For this review, take the finished solid that the model builds, in its own axes (mm). Face numbers are marked on the shaded views. A direction names the side the tool comes from. Give positions to 0.01 mm unless a question says otherwise; leave off trailing zeros. Loops run counter-clockwise (first coordinate to the right, second up) from the corner with the lowest first, then second, coordinate; pieces in that order, holes last. Notation, with made-up numbers: (39, 64) - (87, 64) arc R17 ccw to (87, 82) - close; hole circle Ø5 at (57.5, 20). An arc over 180 degrees is marked (long way). Use CSV: the item, a comma, the result in double quotes. Start each with the question number.
1. Take a section at B-B on y = 0. Give the boundary of the cut face in (x, z).
2. Wall thickness on line 1 (Y direction, x = 0, z = 15.2); line 2 (Y direction, x = 0, z = 9.75); line 3 (X direction, y = 2, z = 15.75): over which ranges is each line inside the solid? List them lowest first.
3. For the marked faces 1, 2 and 3, list the 3-axis set-ups (+Z, -Z, +X, -X, +Y, -Y) from which the entire face can be reached by the end or side of a thin tool; tool diameter is ignored.
4. Take a section at C-C on z = 13. Give the boundary of the cut face in (x, y), plus the area to 3 significant figures.
5. Mouldability with a two-part tool opening along Y and no side actions: class the marked faces 4, 5 and 6 as pulls with the +Y half, pulls with the -Y half, needs draft (parallel to the pull), parting line crosses it, or undercut.
6. Take a section at A-A on x = 0. Give the boundary of the cut face in (y, z), plus the area to 3 significant figures.
7. For pin 1 (2 mm diameter, centred on y = 20.5, z = 7.5, fed in from +X); pin 2 (5 mm diameter, centred on y = -5, z = 11, fed in from +X); pin 3 (8 mm diameter, centred on x = 9.5, z = 6.5, fed in from +Y), all flat-tipped, find the tip position at first contact; note any pin that passes through.
```python
from build123d import *

# Parameters (mm, degrees)
F0_R     = 31
F1_DEPTH = 16
F2_R     = 26
F2_R_2   = 21
F3_DEPTH = 1
F4_R     = 15
F5_DEPTH = 25
F6_W     = 8
F6_H     = 3
F7_DEPTH = 25
F8_R     = 1


with BuildPart() as f1:
    # F0 (on Top) → F1 (new body)
    with BuildSketch(Plane.XY):
        Circle(F0_R)
    extrude(amount=F1_DEPTH)

    # F2 (on face) → F3 (cut)
    with BuildSketch(Plane.XY.offset(16)):
        Circle(F2_R)
        Circle(F2_R_2, mode=Mode.SUBTRACT)
    extrude(amount=-F3_DEPTH, mode=Mode.SUBTRACT)

    # F4 (on face) → F5 (cut)
    with BuildSketch(Plane.XY.offset(16)):
        Circle(F4_R)
    extrude(amount=-F5_DEPTH, mode=Mode.SUBTRACT)

    # F6 (on face) → F7 (cut)
    with BuildSketch(Plane.XY.offset(16)):
        with Locations((0, 15.5)):
            Rectangle(F6_W, F6_H)
    extrude(amount=-F7_DEPTH, mode=Mode.SUBTRACT)

    # F8
    f8_edges = [f1.edges().sort_by_distance(p)[0] for p in [
        (0, -15, 16),
        (-31, 0, 16),
    ]]
    fillet(f8_edges, radius=F8_R)


solid = f1.part
```
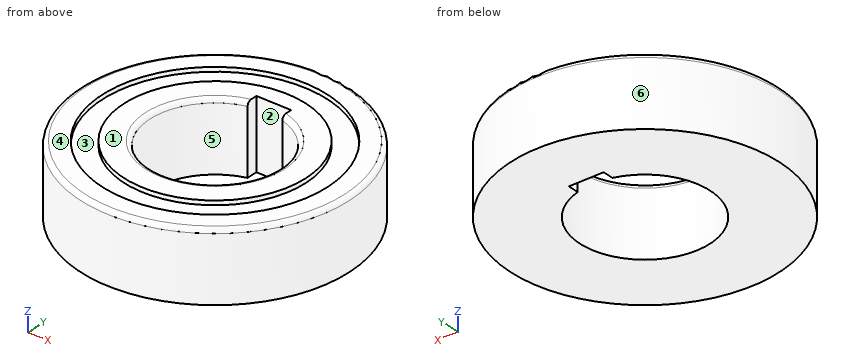
Check result:
1,outline,"(-31, 0) - (-15, 0) - (-15, 15) arc R1 ccw to (-16, 16) - (-21, 16) - (-21, 15) - (-26, 15) - (-26, 16) - (-30, 16) arc R1 ccw to (-31, 15) - close; (15, 0) - (31, 0) - (31, 15) arc R1 ccw to (30, 16) - (26, 16) - (26, 15) - (21, 15) - (21, 16) - (16, 16) arc R1 ccw to (15, 15) - close"
2,line 1,"y = -30.98 to -26, -21 to -15.02, 17 to 21, 26 to 30.98"
2,line 2,"y = -31 to -15, 17 to 31"
2,line 3,"x = -30.6 to -25.92, -20.9 to -15.21, 15.21 to 20.9, 25.92 to 30.6"
3,face 1,"+Z, +X, -X, +Y, -Y"
3,face 2,"+Z, -Z"
3,face 3,"+Z"
4,outline,"circle Ø62 at (0, 0); hole (-4, 14.46) arc R15 ccw (long way) to (4, 14.46) - (4, 17) - (-4, 17) - close"
4,area,"2,290 mm²"
5,face 4,"needs draft"
5,face 5,"undercut"
5,face 6,"parting line crosses it"
6,outline,"(-31, 0) - (-15, 0) - (-15, 15) arc R1 ccw to (-16, 16) - (-21, 16) - (-21, 15) - (-26, 15) - (-26, 16) - (-30, 16) arc R1 ccw to (-31, 15) - close; (17, 0) - (31, 0) - (31, 15) arc R1 ccw to (30, 16) - (26, 16) - (26, 15) - (21, 15) - (21, 16) - (17, 16) - close"
6,area,"469 mm²"
7,pin 1,"stops at x = 24.1"
7,pin 2,"stops at x = 30.9"
7,pin 3,"stops at y = 30.51"
